Source: CAD feature listing. Evaluate the final solid. Frame: model axes, mm. A direction names the side the tool comes from. Give positions to 0.01 mm unless a question says otherwise; leave off trailing zeros. Order: outer loops, then holes, each group sorted by start corner. A loop starts at its lowest first (then second) coordinate and runs counter-clockwise, first axis right, second up. Notation, with made-up numbers: M 37,-32.75 L 42,-32.75 A24 cw 42,-2.75 Z; hole C 33,16.25 d6. An arc over 180 degrees is marked long. Use CSV: the item, a comma, the result in double quotes. Start each with the question number.
1. Section query D-D, the plane y = 15. State how many separate pieces and enclosed holes the cut face has, plus the area to 3 significant figures.
2. Pin query (flat end, axial travel): P1, Ø15, axis at y = 70, z = 44, coming from the -X side; P2, Ø5, axis at y = 17, z = 24, coming from the +X side; P3, Ø1, axis at x = -7.5, y = 27.5, coming from the +Z side. Return the tip coordinate at first contact, or that it passes through.
3. Section query A-A, the plane y = 37.5. Return the cut outline in (x, z).
4. Section query B-B, the plane z = 57.5. Return the cut outline in (x, y).
5. Line query: line 1 along Y through (x, z) = (-1.9, 44); line 2 along Y through (x, z) = (-3.85, 24); line 3 along Z through (x, y) = (-8.5, 67.5). Output: solid intervals per line, ascending. Write a range as [from, to].
6. Reachability of faces 5 (the flat face through (-2, 55, 34)), 6 (the cylindrical face through (-1.479, 65.363, 25.03)), 7 (the flat face through (-9.513, 15.048, -1.025)) from +Z, -Z, +X, -X, +Y, -Y: full face, straight path, thin tool, end or side. Return the list, or none.
7. Mould query, pull axis Z, two halves, no side actions, for faces 1 (the flat face through (0, 23, 34)), 2 (the flat face through (-5, 42, 73)), 3 (the cylindrical face through (-3.986, 72.578, 24.338)), 4 (the cylindrical face through (-1.48, 18.21, 47.5)). Classes: released by +Z, released by -Z, zero draft, split by the parting line, or undercut.
8. Section query C-C, the plane z = 24. Return the cut outline in (x, y), plus the area to 3 significant figures.
Autodesk Inventor part; units mm, degrees
ref_plane "Work Plane2" through (-12.1066, 0, 34) normal (0, 0, 1) x (1, 0, 0)
ref_plane "YZ Plane" through (0, 0, 0) normal (1, 0, 0) x (0, 1, 0)
ref_plane "XZ Plane" through (0, 0, 0) normal (0, 1, 0) x (-1, 0, 0)
sketch "Sketch1" plane through (0, 0, 0) normal (0, 1, 0) x (-1, 0, 0)
  line L0 (0, 0) -> (0, 68)
  line L1 (0, 0) -> (10.6066, -10.6066)
  line L2 (0, 68) -> (10.6066, 78.6066)
  line L3 (5, 63) -> (5, 5)
  line L4 (10.6066, 78.6066) -> (10.6066, 63)
  line L5 (10.6066, -10.6066) -> (10.6066, 5)
  line L6 (10.6066, 63) -> (5, 63)
  line L7 (10.6066, 5) -> (5, 5)
  line L8 (10.6066, 5) -> (12.1066, 5)
  line L9 (12.1066, 5) -> (12.1066, -10.6066)
  line L10 (12.1066, -10.6066) -> (10.6066, -10.6066)
  line L11 (10.6066, -10.6066) -> (10.6066, 5)
  line L12 (10.6066, 63) -> (12.1066, 63)
  line L13 (12.1066, 63) -> (12.1066, 78.6066)
  line L14 (12.1066, 78.6066) -> (10.6066, 78.6066)
  line L15 (10.6066, 78.6066) -> (10.6066, 63)
  dimension "d0" = 68
  dimension "d1" = 15
  dimension "d2" = 135
  dimension "d4" = 15
  dimension "d5" = 135
  dimension "d6" = 5
  dimension "d7" = 5
  dimension "d8" = 5
  dimension "d35" = 1.5
extrude "Extrusion1" add sketch "Sketch1" along normal blind 85
sketch "Sketch2" plane through (0, 0, 68) normal (0.7071, 0, 0.7071) x (0.7071, 0, -0.7071)
  line L0 (-15, 0) -> (0, 0) construction
  line L1 (-7.5, 0) -> (-7.5, 200) construction
  circle A0 centre (-7.5, 70) radius 3.45
  circle A1 centre (-7.5, 15) radius 3.45
  line L2 (-15, 85) -> (0, 85)
  point P0 (48.0833, 0)
  point P1 (-15, 200)
  dimension "d11" = 6.9
  dimension "d12" = 6.9
  dimension "d13" = 15
  dimension "d14" = 15
extrude "Extrusion2" cut sketch "Sketch2" against normal blind 6
sketch "Sketch3" plane through (0, 0, 68) normal (1, 0, 0) x (0, 0, -1)
  ellipse E0 centre (-5.3033, 70) end of major axis (-5.3033, 66.55) minor radius 2.4395 construction
  ellipse E1 centre (73.3033, 70) end of major axis (73.3033, 73.45) minor radius 2.4395 construction
  line L0 (-5.3033, 70) -> (73.3033, 70) construction
  ellipse E2 centre (-5.3033, 15) end of major axis (-5.3033, 11.55) minor radius 2.4395 construction
  ellipse E3 centre (73.3033, 15) end of major axis (73.3033, 18.45) minor radius 2.4395 construction
  line L1 (-5.3033, 15) -> (73.3033, 15) construction
  line L2 (0, 85) -> (68, 85) construction
  line L3 (34, 85) -> (34, 0) construction
  line L4 (63, 0) -> (5, 0) construction
  line L5 (44, 85) -> (44, -115) construction
  line L6 (24, 85) -> (24, -115) construction
  circle A0 centre (44, 70) radius 2.6
  circle A1 centre (24, 70) radius 2.6
  circle A2 centre (24, 15) radius 2.6
  circle A3 centre (44, 15) radius 2.6
  point P0 (68, 0)
  dimension "d17" = 10
  dimension "d18" = 10
  dimension "d19" = 5.2
  dimension "d20" = 5.2
  dimension "d21" = 5.2
  dimension "d22" = 5.2
extrude "Extrusion3" cut sketch "Sketch3" against normal up to next
sketch "Sketch4" plane through (0, 0, 68) normal (1, 0, 0) x (0, 0, -1)
  line L0 (5, 0) -> (5, 85)
  line L1 (63, 0) -> (63, 85)
  line L2 (5, 55) -> (63, 55)
  line L3 (5, 30) -> (63, 30)
  circle A0 centre (24, 70) radius 2.6
  circle A1 centre (24, 15) radius 2.6
  point P0 (68, 0)
  dimension "d25" = 15
  dimension "d26" = 15
extrude "Extrusion4" cut sketch "Sketch4" against normal up to next contours L0 L2 L1 L3
sketch "Sketch5" plane through (0, 0, 68) normal (1, 0, 0) x (0, 0, -1)
  circle A0 centre (24, 70) radius 2.6
  circle A1 centre (24, 70) radius 4.75
  circle A2 centre (44, 70) radius 2.6
  circle A3 centre (44, 70) radius 4.75
  circle A4 centre (24, 15) radius 2.6
  circle A5 centre (24, 15) radius 4.75
  circle A6 centre (44, 15) radius 2.6
  circle A7 centre (44, 15) radius 4.75
  point P0 (68, 0)
  dimension "d29" = 9.5
  dimension "d30" = 9.5
  dimension "d31" = 9.5
  dimension "d32" = 9.5
extrude "Extrusion5" cut sketch "Sketch5" against normal blind 3
ref_plane "Work Plane2" through (-12.1066, 0, 34) normal (0, 0, 1) x (1, 0, 0)
mirror "Mirror2" about plane through (-12.1066, 0, 34) normal (0, 0, 1) of "Extrusion2"
equation "\"d4\" = d1"
equation "\"d5\" = d2"
equation "\"d12\" = d11"
equation "\"d14\" = d13"
equation "\"d20\" = d19"
equation "\"d21\" = d19"
equation "\"d22\" = d19"
equation "\"d30\" = d29"
equation "\"d31\" = d29"
equation "\"d32\" = d29"
properties part number "Z Axis Cover Frame Bottom"
Result set:
1,separate pieces,"3"
1,enclosed holes,"0"
1,area,"395 mm2"
2,P1,"x = -5"
2,P2,"x = -3"
2,P3,"z = 76"
3,outline,"M -12.11,-10.61 L -10.61,-10.61 L 0,0 L 0,5 L -12.11,5 Z; M -12.11,63 L 0,63 L 0,68 L -10.61,78.61 L -12.11,78.61 Z"
4,outline,"M -5,0 L 0,0 L 0,30 L -5,30 Z; M -5,55 L 0,55 L 0,85 L -5,85 Z"
5,line 1,"[0, 10.25], [19.75, 30], [55, 65.25], [74.75, 85]"
5,line 2,"[0, 12.4], [17.6, 30], [55, 67.4], [72.6, 85]"
5,line 3,"[-8.5, -5.47], [-0.01, 5], [63, 68.01], [73.47, 76.5]"
6,face 5,"+X, -X"
6,face 6,"+X"
6,face 7,"none"
7,face 1,"zero draft"
7,face 2,"released by +Z"
7,face 3,"undercut"
7,face 4,"undercut"
8,outline,"M -5,0 L 0,0 L 0,10.25 L -3,10.25 L -3,12.4 L -5,12.4 Z; M -5,17.6 L -3,17.6 L -3,19.75 L 0,19.75 L 0,30 L -5,30 Z; M -5,55 L 0,55 L 0,65.25 L -3,65.25 L -3,67.4 L -5,67.4 Z; M -5,72.6 L -3,72.6 L -3,74.75 L 0,74.75 L 0,85 L -5,85 Z"
8,area,"222 mm2"
